Answer from the drawing. Dimensions are ordinates in mm from the lowest x, y and z of the part. Coordinates: 2 decimals unless noted, no trailing zeros. Order: outer loops, then holes, each group sorted by start corner. A loop starts at its lowest first (then second) coordinate and runs counter-clockwise, first axis right, second up. Notation, with made-up numbers: (-8, 16.25) - (15, 16.25) arc R16 ccw to (15, 21.25) - close; hole circle Ø3 at (19.5, 40.5). An arc over 180 degrees is marked (long way). Use a Markdown table: item, result. Add a question column.
Item 1: The part is cut by section C-C, the plane z = 1.5. State how many separate pieces and enclosed holes the cut face has, then the cut area to 4 significant figures.
Item 2: The part is cut by section A-A, the plane y = 34. Give the vertices of the cut face in (x, z).
Item 3: The part is cut by section D-D, the plane y = 59.5. Give the vertices of the cut face in (x, z).
Item 4: Find the intervals of material crossed by line 1 along Y through (x, z) = (34, 0.8); line 2 along X through (y, z) = (34.5, 1.9); line 3 along Y through (x, z) = (53, 1.2) (1 decimal), in increasing order.
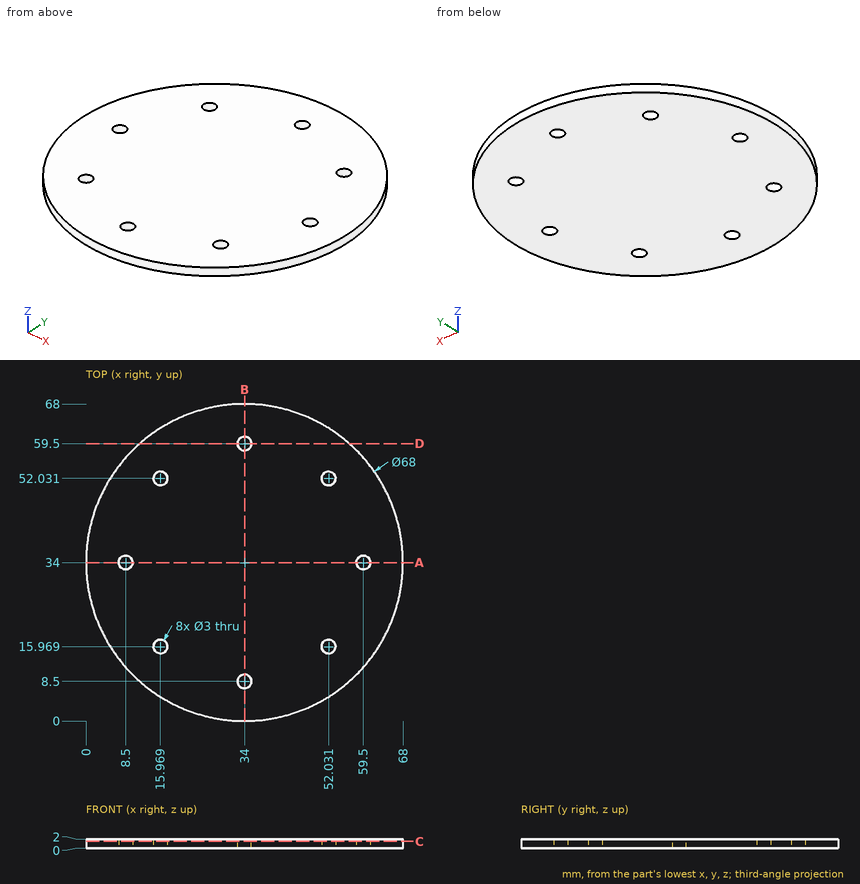
Solution:
| question | item | result |
|---|---|---|
| 1 | separate pieces | 1 |
| 1 | enclosed holes | 8 |
| 1 | area | 3,575 mm2 |
| 2 | outline | (0, 0) - (7, 0) - (7, 2) - (0, 2) - close; (10, 0) - (58, 0) - (58, 2) - (10, 2) - close; (61, 0) - (68, 0) - (68, 2) - (61, 2) - close |
| 3 | outline | (11.51, 0) - (32.5, 0) - (32.5, 2) - (11.51, 2) - close; (35.5, 0) - (56.49, 0) - (56.49, 2) - (35.5, 2) - close |
| 4 | line 1 | y = 0 to 7, 10 to 58, 61 to 68 |
| 4 | line 2 | x = 0 to 7.09, 9.91 to 58.09, 60.91 to 68 |
| 4 | line 3 | y = 5.8 to 14.8, 17.1 to 50.9, 53.2 to 62.2 |
